Part model, mm, in its own coordinate system. A direction names the side the tool comes from. Round coordinates to 2 decimals unless told otherwise and drop trailing zeros. Write each loop counter-clockwise with the first axis right and the second up, starting at its lowest first coordinate (ties: lowest second). Pieces come first, ordered by that corner, then holes. Notation, with made-up numbers: M 66,87 L 118,87 A28 cw 118,105 Z; hole C 42,68 d6. An arc over 180 degrees is marked long. Use a Markdown table: item, result. Add a question column.
1) Slice it at A-A on z = 0. Write the cut outline in (x, y), plus the area to 3 significant figures.
2) Which spindle directions (+Z, -Z, +X, -X, +Y, -Y) get a long thin tool onto all of the face, cutting with end or side? Do faces 4 (the face through (-7.331, 4.93, -62.698)), 5 (the face through (1.208, 4.93, -67.908)), 6 (the face through (47.5, 5, -1)), 7 (the face through (43.939, -14.297, 29.113)), 8 (the face through (47.6, -14.3, 24.6)). Say none if no direction does.
3) Drop flat-ended pins along their axis: P1, Ø4, axis at y = -8, z = 36, coming from the +X side; P2, Ø3, axis at x = 1.5, y = -3, coming from the +Z side; P3, Ø1.5, axis at x = 7.5, y = 4, coming from the +Z side. Give the stop position or say it passes through.
4) Slice it at B-B on x = -27. Write the cut outline in (y, z).
5) Slice it at C-C on x = 30. Write the cut outline in (y, z), plus the area to 3 significant figures.
6) Two-plate mould, pull along Y, no slides. Class faces 1 (the face through (-18, 10, -6)), 2 (the face through (56, 5, -35.262)), 3 (the face through (23.51, 4.93, -68.42)): released by +Y, released by -Y, zero draft, split by the parting line, or undercut.
7) Wall check: probe 1 along Z at (x, y) = (-10.5, 2.5); probe 2 along Z at (x, y) = (1, 4.5); probe 3 along Y at (x, z) = (42.5, -39). Give the ranges that are in metal, low to high.
```python
from build123d import *

# Parameters (mm, degrees)
BOSS_EXTRUDE1_DEPTH               = 10
BOSS_EXTRUDE3_DEPTH               = 10
TAP_DRILL_FOR_M4_TAP1_D           = 3.3
TAP_DRILL_FOR_M4_TAP1_CSINK_D     = 3.35
TAP_DRILL_FOR_M4_TAP1_CSINK_ANGLE = 90
CIRPATTERN1_OUTLINE_W             = 0.025
CIRPATTERN1_OUTLINE_H             = 10
CIRPATTERN1_START                 = -36.401802592
CIRPATTERN1_2_OUTLINE_W           = 14.892514764
CIRPATTERN1_2_OUTLINE_H           = 10
CIRPATTERN1_2_OUTLINE_R           = 1.675
CIRPATTERN1_2_DEPTH               = 10
CIRPATTERN1_START_2               = 23.598197408
CIRPATTERN1_3_OUTLINE_W           = 14.892514764
CIRPATTERN1_3_OUTLINE_H           = 10
CIRPATTERN1_3_OUTLINE_R           = 1.675
CIRPATTERN1_3_DEPTH               = 10
CIRPATTERN1_4_OUTLINE_R           = 1.675
CIRPATTERN1_4_DEPTH               = 1.140104786
CIRPATTERN1_5_OUTLINE_W           = 14.892514764
CIRPATTERN1_5_OUTLINE_H           = 10
CIRPATTERN1_5_OUTLINE_R           = 1.65
CIRPATTERN1_5_DEPTH               = 10
CIRPATTERN1_6_OUTLINE_W           = 14.892514764
CIRPATTERN1_6_OUTLINE_H           = 10
CIRPATTERN1_6_OUTLINE_R           = 1.65
CIRPATTERN1_6_DEPTH               = 10
SKETCH13_R                        = 15.980929879
CUT_EXTRUDE1_DEPTH                = 120.91610231
BOSS_EXTRUDE4_DEPTH               = 29
SKETCH16_R                        = 2
CUT_EXTRUDE2_DEPTH                = 6
SKETCH17_R                        = 2
CUT_EXTRUDE3_DEPTH                = 6


with BuildPart() as part:
    # Sketch2 → Boss-Extrude1 (new body)
    with BuildSketch(Plane(origin=(0, 0, 0), x_dir=(0, 0, -1), z_dir=(0, 1, 0))):
        with BuildLine():
            Line((-58.63620668, -6.560889132), (-77.942286341, -40))
            ThreePointArc((-77.942286341, -40), (-77.942286341, -45), (-73.612159322, -47.5))
            Line((-73.612159322, -47.5), (-35, -47.5))
            Line((-35, -47.5), (-25, -47.5))
            Line((-25, -47.5), (25, -47.5))
            Line((25, -47.5), (35, -47.5))
            Line((35, -47.5), (73.612159322, -47.5))
            ThreePointArc((73.612159322, -47.5), (77.942286341, -45), (77.942286341, -40))
            Line((77.942286341, -40), (58.63620668, -6.560889132))
            Line((58.63620668, -6.560889132), (53.63620668, 2.099364905))
            Line((53.63620668, 2.099364905), (28.63620668, 45.400635095))
            Line((28.63620668, 45.400635095), (23.63620668, 54.060889132))
            Line((23.63620668, 54.060889132), (4.330127019, 87.5))
            ThreePointArc((4.330127019, 87.5), (0, 90), (-4.330127019, 87.5))
            Line((-4.330127019, 87.5), (-23.63620668, 54.060889132))
            Line((-23.63620668, 54.060889132), (-28.63620668, 45.400635095))
            Line((-28.63620668, 45.400635095), (-53.63620668, 2.099364905))
            Line((-53.63620668, 2.099364905), (-58.63620668, -6.560889132))
        make_face()
    extrude(amount=BOSS_EXTRUDE1_DEPTH)

    # Sketch2<7> → Boss-Extrude3 (add)
    with BuildSketch(Plane(origin=(0, 0, 0), x_dir=(0, 0, -1), z_dir=(0, 1, 0))):
        Polygon((58.63620668, -6.560889132), (53.63620668, 2.099364905), (68.63620668, 10.759618943), (73.63620668, 2.099364905), align=None)
        Polygon((23.63620668, 54.060889132), (38.63620668, 62.72114317), (43.63620668, 54.060889132), (28.63620668, 45.400635095), align=None)
    extrude(amount=BOSS_EXTRUDE3_DEPTH)

    # Tap Drill for M4 Tap1 (through all)
    with Locations(Plane(origin=(-30.310889132, 0, 17.5), x_dir=(0.49999999999999517, 0, 0.8660254037844415), z_dir=(-0.8660254037844414, 0, 0.4999999999999951))):
        with Locations((-56.160254038, 5)):
            CounterSinkHole(TAP_DRILL_FOR_M4_TAP1_D / 2, TAP_DRILL_FOR_M4_TAP1_CSINK_D / 2, counter_sink_angle=TAP_DRILL_FOR_M4_TAP1_CSINK_ANGLE)



with BuildPart() as body_2:
    # CirPattern1: read off the stored shape, not the designer's step
    # CirPattern1 outline → CirPattern1 (revolve)
    with BuildSketch(Plane(origin=(55.706980142, 5, 0), x_dir=(1, 0, 0), z_dir=(0, -1, 0))):
        with Locations((1.6625, 28.598197408)):
            Rectangle(CIRPATTERN1_OUTLINE_W, CIRPATTERN1_OUTLINE_H)
        Polygon((1.675, -26.401802592), (1.65, -26.401802592), (1.65, -35.236697806), (1.675, -35.261697806), align=None)
    revolve(axis=Axis((55.706980142, 5, 0), (0, 0, 1)))


with BuildPart() as part_1:
    add(part.part)

    add(body_2.part)  # CirPattern1 2 merges body 2
    # CirPattern1 2 outline → CirPattern1 2 (add)
    with BuildSketch(Plane.XY.offset(CIRPATTERN1_START)):
        with Locations((54.946257382, 5)):
            Rectangle(CIRPATTERN1_2_OUTLINE_W, CIRPATTERN1_2_OUTLINE_H)
        with Locations((55.706980142, 5)):
            Circle(CIRPATTERN1_2_OUTLINE_R, mode=Mode.SUBTRACT)
    extrude(amount=CIRPATTERN1_2_DEPTH)

    # CirPattern1 3 outline → CirPattern1 3 (add)
    with BuildSketch(Plane.XY.offset(CIRPATTERN1_START_2)):
        with Locations((54.946257382, 5)):
            Rectangle(CIRPATTERN1_3_OUTLINE_W, CIRPATTERN1_3_OUTLINE_H)
        with Locations((55.706980142, 5)):
            Circle(CIRPATTERN1_3_OUTLINE_R, mode=Mode.SUBTRACT)
    extrude(amount=CIRPATTERN1_3_DEPTH)

    # CirPattern1 4 outline → CirPattern1 4 (add)
    with BuildSketch(Plane.XY.offset(CIRPATTERN1_START)):
        with Locations((55.706980142, 5)):
            Circle(CIRPATTERN1_4_OUTLINE_R)
    extrude(amount=CIRPATTERN1_4_DEPTH)

    # CirPattern1 5 outline → CirPattern1 5 (add)
    with BuildSketch(Plane(origin=(0, 0, 0), x_dir=(0.500000000000001, 0, -0.866025403784438), z_dir=(0.866025403784438, 0, 0.500000000000001)).offset(CIRPATTERN1_START)):
        with Locations((-54.946257382, 5)):
            Rectangle(CIRPATTERN1_5_OUTLINE_W, CIRPATTERN1_5_OUTLINE_H)
        with Locations((-55.706980142, 5)):
            Circle(CIRPATTERN1_5_OUTLINE_R, mode=Mode.SUBTRACT)
    extrude(amount=CIRPATTERN1_5_DEPTH)

    # CirPattern1 6 outline → CirPattern1 6 (add)
    with BuildSketch(Plane(origin=(0, 0, 0), x_dir=(0.500000000000001, 0, -0.866025403784438), z_dir=(0.866025403784438, 0, 0.500000000000001)).offset(CIRPATTERN1_START_2)):
        with Locations((-54.946257382, 5)):
            Rectangle(CIRPATTERN1_6_OUTLINE_W, CIRPATTERN1_6_OUTLINE_H)
        with Locations((-55.706980142, 5)):
            Circle(CIRPATTERN1_6_OUTLINE_R, mode=Mode.SUBTRACT)
    extrude(amount=CIRPATTERN1_6_DEPTH)

    # Sketch13 → Cut-Extrude1 (cut, through all)
    with BuildSketch(Plane.XZ):
        with Locations(Location((0.00701443, 0.012149349, 0), (0, 0, 270))):
            Circle(SKETCH13_R)
    extrude(amount=-CUT_EXTRUDE1_DEPTH, mode=Mode.SUBTRACT)

    # Sketch15 → Boss-Extrude4 (add)
    with BuildSketch(Plane.XZ):
        Polygon((-3.631756095, 39.600919679), (-3.160458196, 39.433951748), (2.023818696, 37.5973045), (4.027433875, 43.252879291), (-1.628140916, 45.25649447), align=None)
        Polygon((46.137302064, 21.969106104), (46.608599963, 21.802138173), (48.612215142, 27.457712963), (42.956640351, 29.461328142), (40.953025172, 23.805753352), align=None)
    extrude(amount=BOSS_EXTRUDE4_DEPTH)

    # Sketch16 → Cut-Extrude2 (cut)
    with BuildSketch(Plane(origin=(12.06005593, 0, 34.041740653), x_dir=(-0.9425957984699193, 0, 0.3339358631636553), z_dir=(-0.33393586316365526, 0, -0.9425957984699191))):
        with Locations((-34.152554668, -23.871092604)):
            Circle(SKETCH16_R)
        with Locations((-34.152554668, -13.871092604)):
            Circle(SKETCH16_R)
    extrude(amount=-CUT_EXTRUDE2_DEPTH, mode=Mode.SUBTRACT)

    # Sketch17 → Cut-Extrude3 (cut)
    with BuildSketch(Plane(origin=(12.06005593, 0, 34.041740653), x_dir=(-0.9425957984699224, 0, 0.33393586316364626), z_dir=(-0.33393586316364626, 0, -0.9425957984699224))):
        with Locations((14.147445332, -23.871092604)):
            Circle(SKETCH17_R)
        with Locations((14.147445332, -13.871092604)):
            Circle(SKETCH17_R)
    extrude(amount=-CUT_EXTRUDE3_DEPTH, mode=Mode.SUBTRACT)


solid = part_1.part
```
Entries:
| question | item | result |
|---|---|---|
| 1 | outline | M -90,0 L -15.97,0 L -15.97,10 L -90,10 Z; M 15.99,0 L 47.5,0 L 47.5,10 L 15.99,10 Z |
| 1 | area | 1,060 mm^2 |
| 2 | face 4 | -X, +Y, -Y |
| 2 | face 5 | -Z, +Y, -Y |
| 2 | face 6 | +X, +Y, -Y |
| 2 | face 7 | +Z, +X, -Y |
| 2 | face 8 | -Z, +X, -Y |
| 3 | P1 | stops at x = 2.17 |
| 3 | P2 | stops at z = 44.68 |
| 3 | P3 | stops at z = 59.61 |
| 4 | outline | M 0,-39.26 L 10,-39.26 L 10,39.26 L 0,39.26 Z |
| 5 | outline | M 0,-72.17 L 10,-72.17 L 10,72.17 L 0,72.17 Z |
| 5 | area | 1,440 mm^2 |
| 6 | face 1 | released by +Y |
| 6 | face 2 | undercut |
| 6 | face 3 | zero draft |
| 7 | probe 1 | z = -68.79 to -68.19, -48.79 to -12.03, 12.05 to 48.79, 65.38 to 65.98 |
| 7 | probe 2 | z = -68.27 to -67.24, -63.61 to -15.94, 15.96 to 63.09 |
| 7 | probe 3 | y = 0 to 10 |
